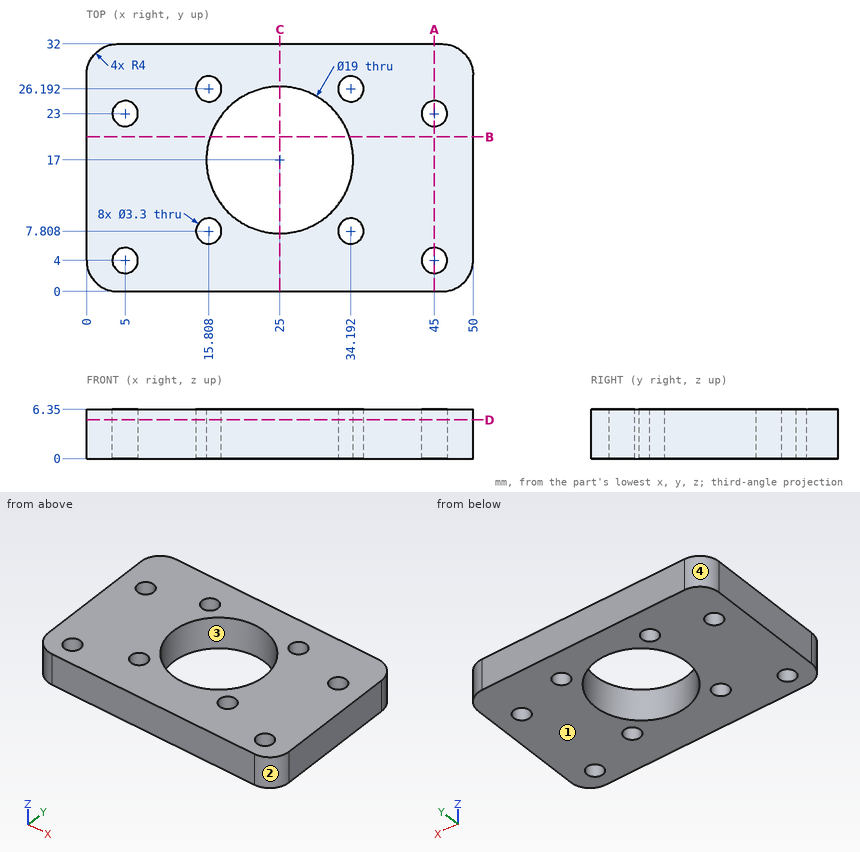
Can you work these out from the drawing? Everything is in mm from the part's minimum corner. Round coordinates to 2 decimals unless told otherwise and drop trailing zeros. Write each loop counter-clockwise with the first axis right and the second up, starting at its lowest first coordinate (ties: lowest second). Pieces come first, ordered by that corner, then holes.
1. Suppose I cut it at B-B (y = 20). List the corners of the cut face in (x, z) for me.
2. Suppose I cut it at A-A (x = 45). List the corners of the cut face in (y, z) for me.
3. Will these pins go through, and if not, where does the flat tip stop? pin 1 Ø2.5 at (x, y) = (45, 23) entering from +Z; pin 2 Ø4 at (x, y) = (36, 22.5) entering from -Z.
4. Suppose I cut it at D-D (z = 5). State how many separate pieces and enclosed holes the cut face has, and give its area (3 significant figures).
5. I need wall thicknesses on L1, parallel to Y at x = 45, z = 4; L2, parallel to Y at x = 25, z = 4; L3, parallel to Y at x = 4, z = 3. Which ranges of each line are inside material? Lowest first, please.
6. If we mould it in two halves opening along X, with no side actions, what happens to the marked faces 1, 2, 3 and 4? For each: released by +X, released by -X, zero draft, split by the parting line, or undercut.
7. Suppose I cut it at C-C (x = 25). List the corners of the cut face in (y, z) for me.
Answer sheet:
1. outline: (0, 0) - (15.99, 0) - (15.99, 6.35) - (0, 6.35) - close; (34.01, 0) - (50, 0) - (50, 6.35) - (34.01, 6.35) - close
2. outline: (0, 0) - (2.35, 0) - (2.35, 6.35) - (0, 6.35) - close; (5.65, 0) - (21.35, 0) - (21.35, 6.35) - (5.65, 6.35) - close; (24.65, 0) - (32, 0) - (32, 6.35) - (24.65, 6.35) - close
3. pin 1: passes through
3. pin 2: stops at z = 0
4. separate pieces: 1
4. enclosed holes: 9
4. area: 1,230 mm2
5. L1: y = 0 to 2.35, 5.65 to 21.35, 24.65 to 32
5. L2: y = 0 to 7.5, 26.5 to 32
5. L3: y = 0 to 2.69, 5.31 to 21.69, 24.31 to 32
6. face 1: zero draft
6. face 2: released by +X
6. face 3: undercut
6. face 4: released by -X
7. outline: (0, 0) - (7.5, 0) - (7.5, 6.35) - (0, 6.35) - close; (26.5, 0) - (32, 0) - (32, 6.35) - (26.5, 6.35) - close
